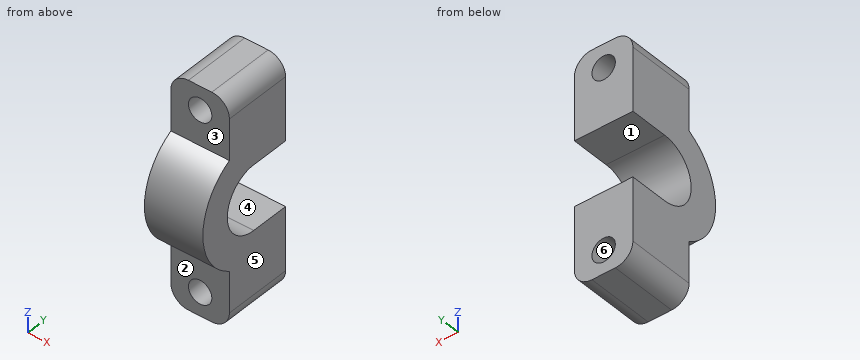
from build123d import *

# Parameters (mm, degrees)
BOSS_EXTRUDE1_DEPTH = 20
CUT_EXTRUDE1_REACH  = 57.463
SKETCH3_R           = 4
FILLET1_R           = 6


with BuildPart() as part:
    # Sketch2 → Boss-Extrude1 (new body)
    with BuildSketch(Plane(origin=(0, 0, 0), x_dir=(0, 0, -1), z_dir=(1, 0, 0))):
        with BuildLine():
            Line((-18.601140422, -10.16), (-38.601140422, -10.16))
            Line((-38.601140422, -10.16), (-38.601140422, 0))
            Line((-38.601140422, 0), (-38.601140422, 13.245))
            Line((-38.601140422, 13.245), (-11.035, 13.245))
            Line((-11.035, 13.245), (-11.035, 0))
            ThreePointArc((-11.035, 0), (0, -11.035), (11.035, 0))
            Line((11.035, 0), (11.035, 13.245))
            Line((11.035, 13.245), (38.601140422, 13.245))
            Line((38.601140422, 13.245), (38.601140422, -10.16))
            Line((38.601140422, -10.16), (18.601140422, -10.16))
            ThreePointArc((18.601140422, -10.16), (0, -21.195), (-18.601140422, -10.16))
        make_face()
    extrude(amount=BOSS_EXTRUDE1_DEPTH)

    # Sketch3 → Cut-Extrude1 (cut, up to next)
    with BuildSketch(Plane(origin=(0, 13.245, 0), x_dir=(1, 0, 0), z_dir=(0, 1, 0)), mode=Mode.PRIVATE) as cut_extrude1_sk1:
        with Locations(Location((10, -30.6, 0), (0, 0, 270))):
            Circle(SKETCH3_R)
    cut_extrude1_tool1 = extrude(cut_extrude1_sk1.sketch, amount=-CUT_EXTRUDE1_REACH, mode=Mode.PRIVATE) & part.part
    # Sketch3 → Cut-Extrude1 (cut, up to next)
    with BuildSketch(Plane(origin=(0, 13.245, 0), x_dir=(1, 0, 0), z_dir=(0, 1, 0)), mode=Mode.PRIVATE) as cut_extrude1_sk2:
        with Locations(Location((10, 30.6, 0), (0, 0, 270))):
            Circle(SKETCH3_R)
    cut_extrude1_tool2 = extrude(cut_extrude1_sk2.sketch, amount=-CUT_EXTRUDE1_REACH, mode=Mode.PRIVATE) & part.part
    add(cut_extrude1_tool1.solids().sort_by_distance((10, 13.245, 30.6))[0], mode=Mode.SUBTRACT)
    add(cut_extrude1_tool2.solids().sort_by_distance((10, 13.245, -30.6))[0], mode=Mode.SUBTRACT)

    # Fillet1
    fillet1_edges = [part.edges().sort_by_distance(p)[0] for p in [
        (0, 1.5425, -38.601140422),
        (0, 1.5425, 38.601140422),
        (20, 1.5425, 38.601140422),
        (20, 1.5425, -38.601140422),
    ]]
    fillet(fillet1_edges, radius=FILLET1_R)


solid = part.part
Source: CAD feature listing. Evaluate the final solid. Frame: model axes, mm. Face numbers are marked on the shaded views. A direction names the side the tool comes from. Give positions to 0.01 mm unless a question says otherwise; leave off trailing zeros. Loops run counter-clockwise (first coordinate to the right, second up) from the corner with the lowest first, then second, coordinate; pieces in that order, holes last. Notation, with made-up numbers: (6.5, 26.5) -> (21.5, 26.5) arc R21 ccw to (21.5, 60.5) -> close; hole circle Ø11 at (-35.5, 81). An arc over 180 degrees is marked (long way). Use a Markdown table: item, result. Add a question column.
1) Section query B-B, the plane x = 10. Return the cut outline in (y, z) (3 decimals), then the cut area to 3 significant figures.
2) Reachability of the marked faces 1, 2 and 3 from +Z, -Z, +X, -X, +Y, -Y: full face, straight path, thin tool, end or side. Return the list, or none.
3) Section query D-D, the plane x = 6.75. Return the cut outline in (y, z) (3 decimals).
4) Pull-direction query (X, two-part tool) for the marked faces 4, 5 and 6; classes: +X half, -X half, draft (parallel to the pull), parting line (faces both ways), or undercut.
5) First-contact query: pin 1 (2 mm diameter, centred on x = 14.5, z = -30.5, fed in from -Y); pin 2 (6 mm diameter, centred on x = 10, y = -17.5, fed in from +Z). Flat tips, straight axial feed; report the tip coordinate or a pass-through.
6) Section query A-A, the plane y = 3. Return the cut outline in (x, z) (3 decimals), then the cut area to 3 significant figures.
7) Section query C-C, the plane z = 30.6. Return the cut outline in (x, y) (3 decimals).
8) Line query: line 1 along X through (y, z) = (2.75, 30.6); line 2 along Z through (x, y) = (6.75, -9); line 3 along Y through (x, z) = (1.5, 35.5) (3 decimals). Output: solid intervals per line, ascending. Write a range as [from, to].
Numbers:
| question | item | result |
|---|---|---|
| 1 | outline | (-10.16, -38.601) -> (13.245, -38.601) -> (13.245, -34.6) -> (-10.16, -34.6) -> close; (-10.16, -26.6) -> (13.245, -26.6) -> (13.245, -11.035) -> (0, -11.035) arc R11.035 cw to (0, 11.035) -> (13.245, 11.035) -> (13.245, 26.6) -> (-10.16, 26.6) -> (-10.16, 18.601) arc R21.195 ccw to (-10.16, -18.601) -> close; (-10.16, 34.6) -> (13.245, 34.6) -> (13.245, 38.601) -> (-10.16, 38.601) -> close |
| 1 | area | 1,240 mm2 |
| 2 | face 1 | +X, -X, +Y |
| 2 | face 2 | -Z, +X, -X, -Y |
| 2 | face 3 | +Z, +X, -X, -Y |
| 3 | outline | (-10.16, -38.601) -> (13.245, -38.601) -> (13.245, -32.932) -> (-10.16, -32.932) -> close; (-10.16, -28.268) -> (13.245, -28.268) -> (13.245, -11.035) -> (0, -11.035) arc R11.035 cw to (0, 11.035) -> (13.245, 11.035) -> (13.245, 28.268) -> (-10.16, 28.268) -> (-10.16, 18.601) arc R21.195 ccw to (-10.16, -18.601) -> close; (-10.16, 32.932) -> (13.245, 32.932) -> (13.245, 38.601) -> (-10.16, 38.601) -> close |
| 4 | face 4 | draft |
| 4 | face 5 | +X half |
| 4 | face 6 | undercut |
| 5 | pin 1 | stops at y = -10.16 |
| 5 | pin 2 | stops at z = 15.46 |
| 6 | outline | (0, -32.601) arc R6 ccw to (6, -38.601) -> (14, -38.601) arc R6 ccw to (20, -32.601) -> (20, -11.035) -> (0, -11.035) -> close; (0, 11.035) -> (20, 11.035) -> (20, 32.601) arc R6 ccw to (14, 38.601) -> (6, 38.601) arc R6 ccw to (0, 32.601) -> close; hole circle Ø8 at (10, -30.6); hole circle Ø8 at (10, 30.6) |
| 6 | area | 971 mm2 |
| 7 | outline | (0, -10.16) -> (6, -10.16) -> (6, 13.245) -> (0, 13.245) -> close; (14, -10.16) -> (20, -10.16) -> (20, 13.245) -> (14, 13.245) -> close |
| 8 | line 1 | x = [0, 6], [14, 20] |
| 8 | line 2 | z = [-38.6, -32.93], [-28.27, -6.39], [6.39, 28.27], [32.93, 38.6] |
| 8 | line 3 | y = [-10.16, 13.245] |
